The figure shows three views and two pictorial views of one solid part (mm, origin at its lowest corner). Answer the questions. A direction names the side the tool comes from. Coordinates: 2 decimals unless noted, no trailing zeros. Order: outer loops, then holes, each group sorted by start corner. A loop starts at its lowest first (then second) coordinate and runs counter-clockwise, first axis right, second up. Notation, with made-up numbers: (43.5, 46.5) - (74.5, 46.5) arc R19 cw to (74.5, 74.5) - close; hole circle Ø5 at (61.5, 44). An arc over 180 degrees is marked (long way). Use one line per item in the form item = value. Start each with the question number.
Item 1: A tool of negligible diameter and unlimited length cuts with its end or side. For the marked faces 1, 2, 3, 4 and 5, from which of +Z, -Z, +X, -X, +Y, -Y can it reach the whole face along a straight path? Write none if from no direction.
Item 2: Each of these flat-tipped pins is pushed along its axis until it touches: pin 1 Ø6 at (y, z) = (28, 12) entering from -X; pin 2 Ø4 at (y, z) = (76, 47) entering from +X; pin 3 Ø1.5 at (x, z) = (42, 52.5) entering from +Y. Where does it stop, or does it pass through?
Item 3: Section C-C, the plane x = 10 is taken. Write down the section's boundary in (y, z).
Item 4: Section D-D, the plane z = 56 is taken. Write down the section's boundary in (x, y), and give its area (3 significant figures).
Item 5: Consider line 1 along Z through (x, y) = (53.5, 167); line 2 along Z through (x, y) = (52, 50); line 3 along Y through (x, z) = (33.5, 45). Determine where each line is inside the solid, lowest interval first. Write a range as [from, to].
Item 6: Section A-A, the plane x = 50 is taken. Write down the section's boundary in (y, z).
Item 7: The mould has two halves that part along Z. Classify the marked faces 6, 7, 8 and 9: released by +Z, released by -Z, zero draft, split by the parting line, or undercut.
Item 8: Section B-B, the plane y = 125 is taken. Write down the section's boundary in (x, z) (3 decimals).
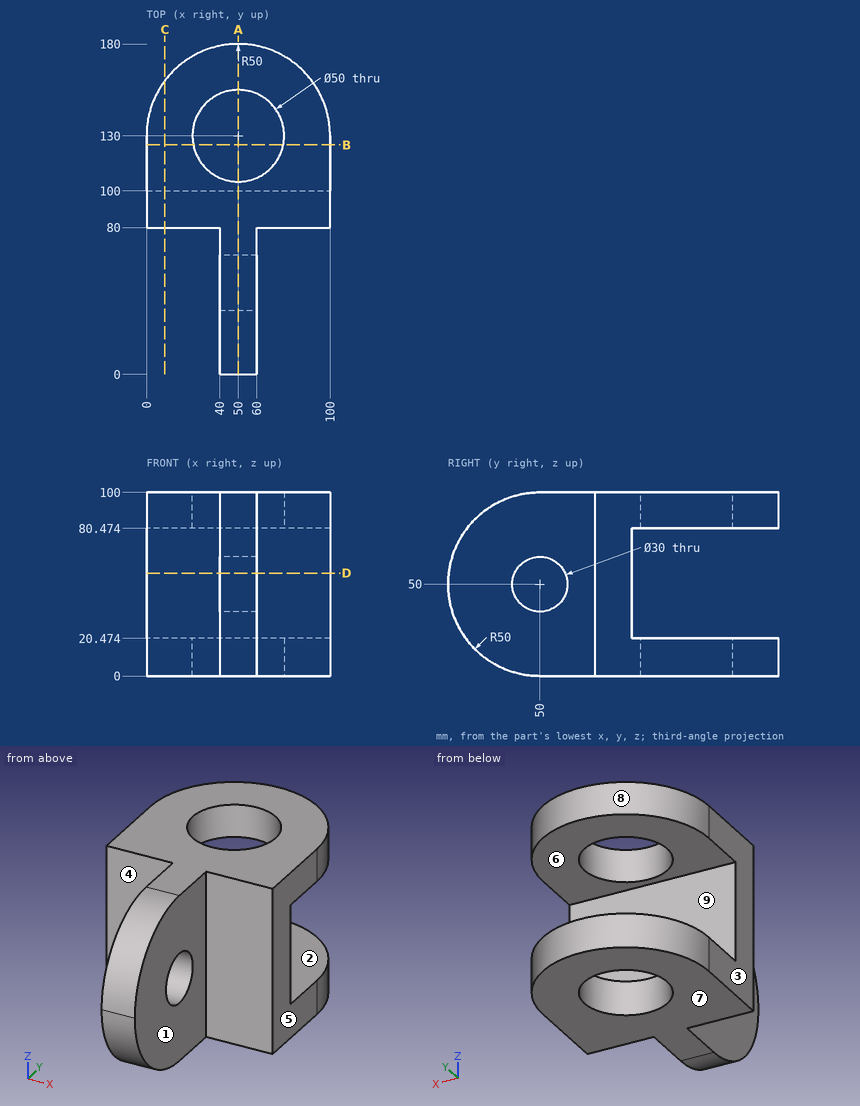
Response:
q1.face_1 = +Z, -Z, +X, -Y
q1.face_2 = +X, -X, +Y
q1.face_3 = +Z, -Z, -X, +Y, -Y
q1.face_4 = +Z, -Z, -X, -Y
q1.face_5 = +Z, -Z, +X, +Y, -Y
q2.pin_1 = 40
q2.pin_2 = 60
q2.pin_3 = 100
q3.outline = (80, 0) - (160, 0) - (160, 20.47) - (100, 20.47) - (100, 80.47) - (160, 80.47) - (160, 100) - (80, 100) - close
q4.outline = (0, 80) - (40, 80) - (40, 63.75) - (60, 63.75) - (60, 80) - (100, 80) - (100, 100) - (0, 100) - close; (40, 0.36) - (60, 0.36) - (60, 36.25) - (40, 36.25) - close
q4.area = 3,040 mm2
q5.line_1 = [0, 20.47], [80.47, 100]
q5.line_2 = [0, 35], [65, 100]
q5.line_3 = [80, 100]
q6.outline = (50, 0) - (105, 0) - (105, 20.47) - (100, 20.47) - (100, 80.47) - (105, 80.47) - (105, 100) - (50, 100) arc R50 ccw to start; (155, 0) - (180, 0) - (180, 20.47) - (155, 20.47) - close; (155, 80.47) - (180, 80.47) - (180, 100) - (155, 100) - close; hole circle Ø30 at (50, 50)
q7.face_6 = undercut
q7.face_7 = released by -Z
q7.face_8 = zero draft
q7.face_9 = undercut
q8.outline = (0, 0) - (25.505, 0) - (25.505, 20.474) - (0, 20.474) - close; (0, 80.474) - (25.505, 80.474) - (25.505, 100) - (0, 100) - close; (74.495, 0) - (100, 0) - (100, 20.474) - (74.495, 20.474) - close; (74.495, 80.474) - (100, 80.474) - (100, 100) - (74.495, 100) - close
